Geometry: final body of the model. Coordinates: model frame, mm. A direction names the side the tool comes from. Give positions to 0.01 mm unless a question says otherwise; leave off trailing zeros. Loops run counter-clockwise (first coordinate to the right, second up) from the corner with the lowest first, then second, coordinate; pieces in that order, holes last. Notation, with made-up numbers: (-19, 73) -> (10, 73) arc R29 ccw to (10, 111) -> close; hole circle Ø11 at (-36, -0.75). An arc over 180 degrees is marked (long way). One line per item, written item: value. Start each with the question number.
from build123d import *

# Parameters (mm, degrees)
SKETCH_1_W          = 50
SKETCH_1_H          = 20
EXTRUDE_1_DEPTH     = 3
SKETCH_3_R          = 5
SKETCH_3_W          = 30
SKETCH_3_H          = 8.678040074
CUT_EXTRUDE_1_DEPTH = 3
SKETCH_4_W          = 2
SKETCH_4_H          = 3
EXTRUDE_2_DEPTH     = 1
FILLET_1_R          = 1
SKETCH_5_W          = 2
SKETCH_5_H          = 3
EXTRUDE_3_DEPTH     = 1
FILLET_2_R          = 1


with BuildPart() as part:
    # 스케치1 → 보스-돌출1 (new body)
    with BuildSketch(Plane.XY):
        Rectangle(SKETCH_1_W, SKETCH_1_H)
    extrude(amount=-EXTRUDE_1_DEPTH)

    # 스케치3 → 컷-돌출1 (cut)
    with BuildSketch(Plane.XY):
        with Locations((-15, 0)):
            Circle(SKETCH_3_R)
        with Locations((15, 0)):
            Circle(SKETCH_3_R)
        Rectangle(SKETCH_3_W, SKETCH_3_H)
    extrude(amount=-CUT_EXTRUDE_1_DEPTH, mode=Mode.SUBTRACT)

    # 스케치4 → 보스-돌출2 (add)
    with BuildSketch(Plane.XZ.offset(-4.339020037)):
        with Locations((-11.515466821, -1.5)):
            Rectangle(SKETCH_4_W, SKETCH_4_H)
        with Locations((11.515466821, -1.5)):
            Rectangle(SKETCH_4_W, SKETCH_4_H)
    extrude(amount=EXTRUDE_2_DEPTH)

    # 필렛1
    fillet_1_edges = [part.edges().sort_by_distance(p)[0] for p in [
        (12.515466821, 3.339020037, -1.5),
        (10.515466821, 3.339020037, -1.5),
        (-10.515466821, 3.339020037, -1.5),
        (-12.515466821, 3.339020037, -1.5),
    ]]
    fillet(fillet_1_edges, radius=FILLET_1_R - 0.0001)  # a hair under: the kernel refuses the full size

    # 스케치5 → 보스-돌출3 (add)
    with BuildSketch(Plane(origin=(0, -4.339020037, 0), x_dir=(1, 0, 0), z_dir=(0, 1, 0))):
        with Locations((-11.515466821, 1.5)):
            Rectangle(SKETCH_5_W, SKETCH_5_H)
    extrude(amount=EXTRUDE_3_DEPTH)

    # 필렛2
    fillet_2_edges = [part.edges().sort_by_distance(p)[0] for p in [
        (-12.515466821, -3.339020037, -1.5),
        (-10.515466821, -3.339020037, -1.5),
    ]]
    fillet(fillet_2_edges, radius=FILLET_2_R - 0.0001)  # a hair under: the kernel refuses the full size


solid = part.part
Item 1: Access query for faces 5 (the face through (-10.82, -3.62, -1.52)), 6 (the face through (25, 0, -1)). Directions: +Z, -Z, +X, -X, +Y, -Y. A direction counts if a zero-diameter tool reaches every point of the face in a straight line with its end or side. Return the directions, or none.
Item 2: Section A-A, the plane y = 0. Output: boundary loops of the cut face in (x, z).
Item 3: Pin query (flat end, axial travel): pin 1 (10 mm diameter, centred on x = 19, y = 6.5, fed in from +Z). Return the tip coordinate at first contact, or that it passes through.
Item 4: Mould query, pull axis Y, two halves, no side actions, for faces 1 (the face through (0, 10, -1)), 2 (the face through (20, 0, -1)), 3 (the face through (0, -5, -3)), 4 (the face through (0, -10, -1)). Classes: pulls with the +Y half, pulls with the -Y half, needs draft (parallel to the pull), parting line crosses it, or undercut.
Item 5: Section C-C, the plane x = 1.5. Output: boundary loops of the cut face in (y, z).
Item 6: Ray query, line 1 along Y through (x, z) = (-5, -0.05); line 2 along X through (y, z) = (4.5, -0.45); line 3 along Y through (x, z) = (-17, -1.1). Return the intervals inside material, ascending. Write a range as [from, to].
Geometry check:
1. face 5: +Z, -Z
1. face 6: +Z, -Z, +X, +Y, -Y
2. outline: (-25, -3) -> (-20, -3) -> (-20, 0) -> (-25, 0) -> close; (20, -3) -> (25, -3) -> (25, 0) -> (20, 0) -> close
3. pin 1: stops at z = 0
4. face 1: pulls with the +Y half
4. face 2: undercut
4. face 3: needs draft
4. face 4: pulls with the -Y half
5. outline: (-10, -3) -> (-4.34, -3) -> (-4.34, 0) -> (-10, 0) -> close; (4.34, -3) -> (10, -3) -> (10, 0) -> (4.34, 0) -> close
6. line 1: y = [-10, -4.34], [4.34, 10]
6. line 2: x = [-25, -17.18], [-12.82, 12.82], [17.18, 25]
6. line 3: y = [-10, -4.58], [4.58, 10]
